Build history of the part. All positions in model axes, mm. A direction names the side the tool comes from. Round coordinates to 2 decimals unless told otherwise and drop trailing zeros. Write each loop counter-clockwise with the first axis right and the second up, starting at its lowest first coordinate (ties: lowest second). Pieces come first, ordered by that corner, then holes.
1) Wall check: probe 1 along Y at (x, z) = (2, 0.85); probe 2 along X at (y, z) = (12, 1.35); probe 3 along X at (y, z) = (-9.5, -2.55). Give the ranges that are in metal, low to high.
2) Flat gauge pins, fed straight in: pin 1 (1.8 mm diameter, centred on x = 0, z = 1, fed in from +Y); pin 2 (5 mm diameter, centred on x = -1.5, y = -13, fed in from -Z); pin 3 (3 mm diameter, centred on x = 6.5, z = 1.5, fed in from -Y); pin 4 (1 mm diameter, centred on y = 14, z = -2, fed in from +X). Where does each tip first touch, or does it go through?
3) Saw through at C-C (z = 1.8). Write the cut outline in (x, y), plus the area to 3 significant figures.
4) Pull direction X, two halves, no side cores. Call faces 3 (the flat face through (0, 13.5, 0)), 4 (the flat face through (11, -11, 3)), 5 (the cylindrical face through (23.846, 7.509, 0.042)): +X half, -X half, draft (parallel to the pull), parting line (faces both ways), or undercut.
5) Saw through at D-D (y = -16.5). Write the cut outline in (x, z), plus the area to 3 significant figures.
6) Which spindle directions (+Z, -Z, +X, -X, +Y, -Y) get a long thin tool onto all of the face, cutting with end or side? Do faces 1 (the flat face through (11, -11, -3)), 2 (the flat face through (0, -13.5, 0)). Say none if no direction does.
7) Saw through at B-B (y = 0). Write the cut outline in (x, z).
8) Saw through at A-A (x = -3). Write the cut outline in (y, z).
from build123d import *

# Parameters (mm, degrees)
SKETCH1_R           = 25
BOSS_EXTRUDE1_DEPTH = 3
SKETCH2_R           = 1
CUT_EXTRUDE1_DEPTH  = 36.860842154
FILLET1_R           = 1


with BuildPart() as part:
    # Sketch1 → Boss-Extrude1 (new, symmetric)
    with BuildSketch(Plane.XY):
        Circle(SKETCH1_R)
        Polygon((-15.588457268, 0), (-7.794228634, -13.5), (7.794228634, -13.5), (15.588457268, 0), (7.794228634, 13.5), (-7.794228634, 13.5), align=None, mode=Mode.SUBTRACT)
    extrude(amount=BOSS_EXTRUDE1_DEPTH, both=True)

    # Sketch2 → Cut-Extrude1 (cut, through all)
    with BuildSketch(Plane.XY.offset(3)):
        with Locations((-7.794228634, 13.5)):
            Circle(SKETCH2_R)
        with Locations((7.794228634, 13.5)):
            Circle(SKETCH2_R)
        with Locations((-15.588457268, 0)):
            Circle(SKETCH2_R)
        with Locations((-7.794228634, -13.5)):
            Circle(SKETCH2_R)
        with Locations((7.794228634, -13.5)):
            Circle(SKETCH2_R)
        with Locations((15.588457268, 0)):
            Circle(SKETCH2_R)
    extrude(amount=-CUT_EXTRUDE1_DEPTH, mode=Mode.SUBTRACT)

    # Fillet1
    fillet1_edges = [part.edges().sort_by_distance(p)[0] for p in [
        (-6.794228634, 13.5, 0),
        (6.794228634, 13.5, 0),
        (15.088457268, 0.866025404, 0),
        (8.294228634, -12.633974596, 0),
        (-6.794228634, -13.5, 0),
        (-15.088457268, -0.866025404, 0),
        (15.088457268, -0.866025404, 0),
        (6.794228634, -13.5, 0),
        (-8.294228634, -12.633974596, 0),
        (-15.088457268, 0.866025404, 0),
        (8.294228634, 12.633974596, 0),
        (-8.294228634, 12.633974596, 0),
    ]]
    fillet(fillet1_edges, radius=FILLET1_R)


solid = part.part
Evaluation:
1. probe 1: y = -24.92 to -13.5, 13.5 to 24.92
1. probe 2: x = -21.93 to -8.66, 8.66 to 21.93
1. probe 3: x = -23.12 to -10.1, 10.1 to 23.12
2. pin 1: stops at y = 25
2. pin 2: stops at z = -3
2. pin 3: stops at y = -24.49
2. pin 4: stops at x = 21.04
3. outline: circle Ø50 at (0, 0); hole (-15.59, -1) arc R1 cw to (-14.72, -1.5) - (-8.66, -12) arc R1 cw to (-8.66, -13) arc R1 ccw to (-6.93, -14) arc R1 cw to (-6.06, -13.5) - (6.06, -13.5) arc R1 cw to (6.93, -14) arc R1 ccw to (8.66, -13) arc R1 cw to (8.66, -12) - (14.72, -1.5) arc R1 cw to (15.59, -1) arc R1 ccw to (15.59, 1) arc R1 cw to (14.72, 1.5) - (8.66, 12) arc R1 cw to (8.66, 13) arc R1 ccw to (6.93, 14) arc R1 cw to (6.06, 13.5) - (-6.06, 13.5) arc R1 cw to (-6.93, 14) arc R1 ccw to (-8.66, 13) arc R1 cw to (-8.66, 12) - (-14.72, 1.5) arc R1 cw to (-15.59, 1) arc R1 ccw to start
3. area: 1,320 mm2
4. face 3: undercut
4. face 4: draft
4. face 5: parting line
5. outline: (-18.78, -3) - (18.78, -3) - (18.78, 3) - (-18.78, 3) - close
5. area: 225 mm2
6. face 1: -Z, +X, -X, +Y, -Y
6. face 2: +Z, -Z
7. outline: (-25, -3) - (-16.59, -3) - (-16.59, 3) - (-25, 3) - close; (16.59, -3) - (25, -3) - (25, 3) - (16.59, 3) - close
8. outline: (-24.82, -3) - (-13.5, -3) - (-13.5, 3) - (-24.82, 3) - close; (13.5, -3) - (24.82, -3) - (24.82, 3) - (13.5, 3) - close
